```python
from build123d import *

# Parameters (mm, degrees)
F0_W     = 254
F0_H     = 161.29
F1_DEPTH = 7.9375
F2_W     = 254
F2_H     = 7.9375
F3_DEPTH = 254
F6_W     = 7.9375
F6_H     = 153.3525
F7_DEPTH = 254
F9_DEPTH = 206.09914
F10_R    = 6.35


with BuildPart() as f1:
    # F0 (on Front) → F1 (new body)
    with BuildSketch(Plane.XZ):
        Rectangle(F0_W, F0_H)
    extrude(amount=F1_DEPTH)

    # F2 (on face) → F3 (join)
    with BuildSketch(Plane.XZ.offset(7.9375)):
        with Locations((0, 76.67625)):
            Rectangle(F2_W, F2_H)
    extrude(amount=F3_DEPTH)

    # F6 (on face) → F7 (join, through all)
    with BuildSketch(Plane.XZ.offset(7.9375)):
        with Locations((-75.12939, -3.96875)):
            Rectangle(F6_W, F6_H)
        with Locations((75.12939, -3.96875)):
            Rectangle(F6_W, F6_H)
    extrude(amount=F7_DEPTH)

    # F8 (on face) → F9 (cut, through all)
    with BuildSketch(Plane(origin=(-79.09814, 0, 0), x_dir=(0, -1, 0), z_dir=(-1, 0, 0))):
        Polygon((261.9375, -80.645), (261.9375, 34.6075), (46.0375, -80.645), align=None)
    extrude(amount=-F9_DEPTH, mode=Mode.SUBTRACT)

    # F10
    f10_edges = [f1.edges().sort_by_distance(p)[0] for p in [
        (-127, -261.9375, 76.67625),
        (127, -261.9375, 76.67625),
    ]]
    fillet(f10_edges, radius=F10_R)


solid = f1.part
```
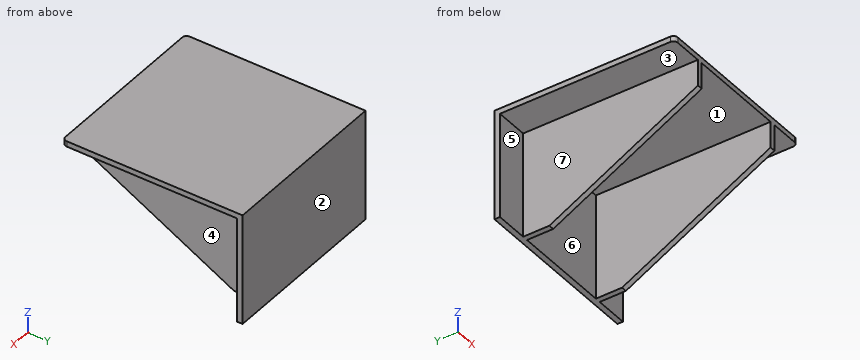
Source: CAD feature listing. Evaluate the final solid. Frame: model axes, mm. Face numbers are marked on the shaded views. A direction names the side the tool comes from. Give positions to 0.01 mm unless a question says otherwise; leave off trailing zeros. Write each loop counter-clockwise with the first axis right and the second up, starting at its lowest first coordinate (ties: lowest second). Pieces come first, ordered by that corner, then holes.
1. First-contact query: pin 1 (1 mm diameter, centred on y = -141, z = -21, fed in from -X); pin 2 (1 mm diameter, centred on x = 55.5, y = -142, fed in from -Z); pin 3 (24 mm diameter, centred on x = -96, z = -4.5, fed in from -Y). Flat tips, straight axial feed; report the tip coordinate or a pass-through.
2. Access query for the marked faces 1, 2 and 3. Directions: +Z, -Z, +X, -X, +Y, -Y. A direction counts if a zero-diameter tool reaches every point of the face in a straight line with its end or side. Return the directions, or none.
3. Section query C-C (x = -75). Return the cut outline in (y, z) (1 decimal), then the cut area to 3 significant figures.
4. Section query B-B (z = 47). Return the cut outline in (x, y), then the cut area to 3 significant figures.
5. Material intervals for line 1 along X through (y, z) = (-118.5, 42); line 2 along Y through (x, z) = (71, -47); line 3 along Z through (x, y) = (111, -104.5) (1 decimal), sorted ascending.
6. Pull-direction query (X, two-part tool) for the marked faces 4, 5, 6 and 7; classes: +X half, -X half, draft (parallel to the pull), parting line (faces both ways), or undercut.
7. Section query D-D (x = -20.5). Return the cut outline in (y, z) (1 decimal), then the cut area to 3 significant figures.
8. Section query A-A (y = -20.5). Return the cut outline in (x, z) (1 decimal), then the cut area to 3 significant figures.
Output values:
1. pin 1: stops at x = -79.1
1. pin 2: stops at z = 72.71
1. pin 3: stops at y = -7.94
2. face 1: -Z, -Y
2. face 2: +Z, -Z, +X, -X, +Y
2. face 3: -Z, -X, -Y
3. outline: (-261.9, 34.6) - (-46, -80.6) - (0, -80.6) - (0, 80.6) - (-261.9, 80.6) - close
3. area: 29,800 mm2
4. outline: (-127, -7.94) - (-79.1, -7.94) - (-79.1, -261.94) - (-71.16, -261.94) - (-71.16, -7.94) - (71.16, -7.94) - (71.16, -261.94) - (79.1, -261.94) - (79.1, -7.94) - (127, -7.94) - (127, 0) - (-127, 0) - close
4. area: 6,050 mm2
5. line 1: x = -79.1 to -71.16, 71.16 to 79.1
5. line 2: y = -7.94 to 0
5. line 3: z = 72.7 to 80.6
6. face 4: +X half
6. face 5: draft
6. face 6: undercut
6. face 7: -X half
7. outline: (-261.9, 72.7) - (-7.9, 72.7) - (-7.9, -80.6) - (0, -80.6) - (0, 80.6) - (-261.9, 80.6) - close
7. area: 3,300 mm2
8. outline: (-127, 72.7) - (-79.1, 72.7) - (-79.1, -80.6) - (-71.2, -80.6) - (-71.2, 72.7) - (71.2, 72.7) - (71.2, -80.6) - (79.1, -80.6) - (79.1, 72.7) - (127, 72.7) - (127, 80.6) - (-127, 80.6) - close
8. area: 4,450 mm2
